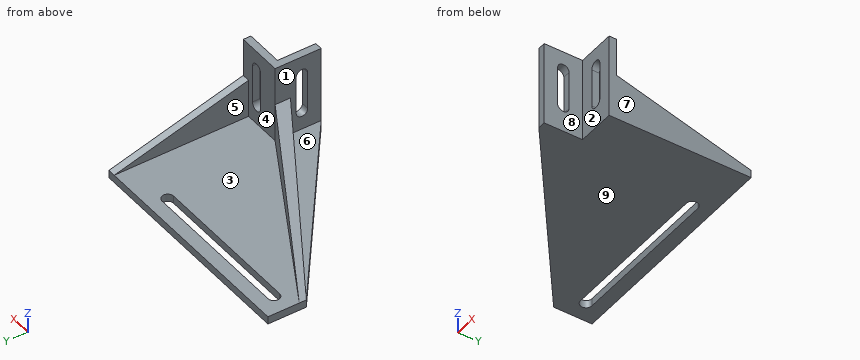
```python
from build123d import *

# Parameters (mm, degrees)
SKETCH_W             = 2
SKETCH_H             = 20
PAD_DEPTH            = 10
POCKET_DEPTH         = 2
SKETCH003_W          = 2
SKETCH003_H          = 20
PAD001_DEPTH         = 10
PAD001_DEPTH_BACK    = 2
POCKET001_DEPTH      = 2.001
PAD002_DEPTH         = 2
PAD003_DEPTH         = 10
PAD003_DEPTH_BACK    = 29
PAD004_DEPTH         = 10
POCKET002_DEPTH      = 2
POCKET002_DEPTH_BACK = -8
POCKET003_DEPTH      = 20.001
POCKET004_DEPTH      = 20.001
POCKET005_DEPTH      = 2.001


with BuildPart() as part:
    # Sketch → Pad (new body)
    with BuildSketch(Plane.XZ):
        with Locations((-1, 10)):
            Rectangle(SKETCH_W, SKETCH_H)
    extrude(amount=PAD_DEPTH)

    # Sketch002 → Pocket (cut)
    with BuildSketch(Plane.YZ):
        with BuildLine():
            ThreePointArc((-3.5, 15), (-5, 16.5), (-6.5, 15))
            Line((-6.5, 15), (-6.5, 5))
            ThreePointArc((-6.5, 5), (-5, 3.5), (-3.5, 5))
            Line((-3.5, 15), (-3.5, 5))
        make_face()
    extrude(amount=-POCKET_DEPTH, mode=Mode.SUBTRACT)

    # Sketch003 → Pad001 (join, two sides)
    with BuildSketch(Plane.YZ) as pad001_sk:
        with Locations((1, 10)):
            Rectangle(SKETCH003_W, SKETCH003_H)
    extrude(amount=PAD001_DEPTH)
    extrude(pad001_sk.sketch, amount=-PAD001_DEPTH_BACK)

    # Sketch001 → Pocket001 (cut, through all)
    with BuildSketch(Plane.XZ):
        with BuildLine():
            ThreePointArc((6.5, 15), (5, 16.5), (3.5, 15))
            Line((3.5, 15), (3.5, 5))
            ThreePointArc((3.5, 5), (5, 3.5), (6.5, 5))
            Line((6.5, 15), (6.5, 5))
        make_face()
    extrude(amount=-POCKET001_DEPTH, mode=Mode.SUBTRACT)

    # Sketch004 → Pad002 (join)
    with BuildSketch(Plane.XY):
        Polygon((-50, 37), (10, 37), (10, 0), (0, 0), (0, -10), (-2, -10), (-50, 27), align=None)
    extrude(amount=-PAD002_DEPTH)

    # Sketch005 → Pad003 (join, two sides)
    with BuildSketch(Plane.XZ) as pad003_sk:
        Polygon((-2, 0), (-50, 0), (-2, 10), align=None)
    extrude(amount=PAD003_DEPTH)
    extrude(pad003_sk.sketch, amount=-PAD003_DEPTH_BACK)

    # Sketch006 → Pad004 (join)
    with BuildSketch(Plane.YZ):
        Polygon((2, 10), (2, 0), (37, 0), align=None)
    extrude(amount=PAD004_DEPTH)

    # Sketch007 → Pocket002 (cut, two sides)
    with BuildSketch(Plane.YZ) as pocket002_sk:
        Polygon((2, 10), (2, 0), (37, 0), align=None)
    extrude(amount=-POCKET002_DEPTH, mode=Mode.SUBTRACT)
    extrude(pocket002_sk.sketch, amount=-POCKET002_DEPTH_BACK, mode=Mode.SUBTRACT)

    # Sketch008 → Pocket003 (cut, through all)
    with BuildSketch(Plane.XY):
        Polygon((-50, 27), (-2, -2), (-2, -12), (-50, -12), align=None)
    extrude(amount=POCKET003_DEPTH, mode=Mode.SUBTRACT)

    # Sketch009 → Pocket004 (cut, through all)
    with BuildSketch(Plane.XY):
        Polygon((-2, 2), (-2, 37), (-50, 37), (-50, 28.830978), align=None)
    extrude(amount=POCKET004_DEPTH, mode=Mode.SUBTRACT)

    # Sketch010 → Pocket005 (cut, through all)
    with BuildSketch(Plane.XY):
        with BuildLine():
            ThreePointArc((-45, 33.5), (-46.5, 32), (-45, 30.5))
            Line((-45, 30.5), (-5, 30.5))
            ThreePointArc((-5, 30.5), (-3.5, 32), (-5, 33.5))
            Line((-45, 33.5), (-5, 33.5))
        make_face()
    extrude(amount=-POCKET005_DEPTH, mode=Mode.SUBTRACT)


solid = part.part
```
Geometry: final body of the model. Coordinates: model frame, mm. Face numbers are marked on the shaded views. A direction names the side the tool comes from. Coordinates: 2 decimals unless noted, no trailing zeros. Order: outer loops, then holes, each group sorted by start corner. A loop starts at its lowest first (then second) coordinate and runs counter-clockwise, first axis right, second up. Notation, with made-up numbers: M 24,2 L 39,2 A15 ccw 39,20 Z; hole C 2.25,63.5 d4. An arc over 180 degrees is marked long. Answer in a Markdown table with one row per item. Add a question column.
Q1. Contact query for flat-ended pins moving along their axis: P1, Ø1.6, axis at y = 0.5, z = 11, coming from the -X side; P2, Ø12, axis at x = -33, z = 5.5, coming from the +Y side; P3, Ø1.6, axis at x = -1.5, z = 9, coming from the +Y side; P4, Ø0.6, axis at x = -17, z = -0.5, coming from the -Y side. Output: stop coordinate, or through.
Q2. Section query B-B on x = 5. Return the cut outline in (y, z).
Q3. Section query C-C on y = -5. Return the cut outline in (x, z).
Q4. Mould query, pull axis X, two halves, no side actions, for the marked faces 1, 2, 3 and 4. Classes: released by +X, released by -X, zero draft, split by the parting line, or undercut.
Q5. Section query D-D on y = 24.5. Return the cut outline in (x, z), and give its area (3 significant figures).
Q6. Section query A-A on z = 13.5. Return the cut outline in (x, y), and give its area (3 significant figures).
Q7. Line query: L1, parallel to Z at x = -12, y = 26; L2, parallel to Y at x = 1, z = -0.25; L3, parallel to Y at x = 3, z = 5.75. Output: solid intervals per line, ascending.
Q8. Reachability of the marked faces 5, 6, 7, 8 and 9 from +Z, -Z, +X, -X, +Y, -Y: full face, straight path, thin tool, end or side. Return the list, or none.
Completed:
| question | item | result |
|---|---|---|
| 1 | P1 | stops at x = -2 |
| 1 | P2 | stops at y = 37 |
| 1 | P3 | stops at y = 2.17 |
| 1 | P4 | stops at y = 1.33 |
| 2 | outline | M 0,-2 L 37,-2 L 37,0 L 2,0 L 2,3.5 L 0,3.5 Z; M 0,16.5 L 2,16.5 L 2,20 L 0,20 Z |
| 3 | outline | M -8.49,-2 L 0,-2 L 0,3.5 L -2,3.5 L -2,0 L -8.49,0 Z; M -2,16.5 L 0,16.5 L 0,20 L -2,20 Z |
| 4 | face 1 | released by -X |
| 4 | face 2 | zero draft |
| 4 | face 3 | undercut |
| 4 | face 4 | undercut |
| 5 | outline | M -46.76,-2 L 10,-2 L 10,3.57 L 8,3.57 L 8,0 L -42.25,0 L -42.25,1.61 L -45.86,0.86 L -45.86,0 L -46.76,0 Z |
| 5 | area | 125 mm2 |
| 6 | outline | M -2,-10 L 0,-10 L 0,-6.5 L -2,-6.5 Z; M -2,-3.5 L 0,-3.5 L 0,0 L 3.5,0 L 3.5,2 L -2,2 Z; M 6.5,0 L 10,0 L 10,2 L 6.5,2 Z |
| 6 | area | 32.0 mm2 |
| 7 | L1 | z = -2 to 0 |
| 7 | L2 | y = 0 to 37 |
| 7 | L3 | y = 0 to 2 |
| 8 | face 5 | +Z, +Y |
| 8 | face 6 | +Z, -X, -Y |
| 8 | face 7 | +Z, -Z, +X, +Y, -Y |
| 8 | face 8 | +Z, -Z, +X, -Y |
| 8 | face 9 | -Z, +X, -X, +Y, -Y |
